```python
from build123d import *

# Parameters (mm, degrees)
F0_W     = 50
F0_H     = 50
F1_DEPTH = 15
F3_DEPTH = 60
F5_DEPTH = 5
F6_W     = 30
F6_H     = 5.4
F7_DEPTH = 30


with BuildPart() as f1:
    # F0 (on Top) → F1 (new body)
    with BuildSketch(Plane.XY):
        with Locations((25, -25)):
            Rectangle(F0_W, F0_H)
    extrude(amount=F1_DEPTH)

    # F2 (on face) → F3 (join)
    with BuildSketch(Plane.XY.offset(15)):
        Polygon((15, -30), (15, -50), (35, -50), (35, -30), (25, -17.510004), align=None)
    extrude(amount=F3_DEPTH)

    # F4 (on face) → F5 (cut)
    with BuildSketch(Plane(origin=(0, 0, 0), x_dir=(1, 0, 0), z_dir=(0, 0, -1))):
        Polygon((35, 50), (15, 50), (15, 30), (25, 17.510004), (35, 30), align=None)
    extrude(amount=-F5_DEPTH, mode=Mode.SUBTRACT)

    # F6 (on face) → F7 (cut)
    with BuildSketch(Plane.YZ.offset(50)):
        with Locations((-15, 7.7)):
            Rectangle(F6_W, F6_H)
    extrude(amount=-F7_DEPTH, mode=Mode.SUBTRACT)


solid = f1.part
```
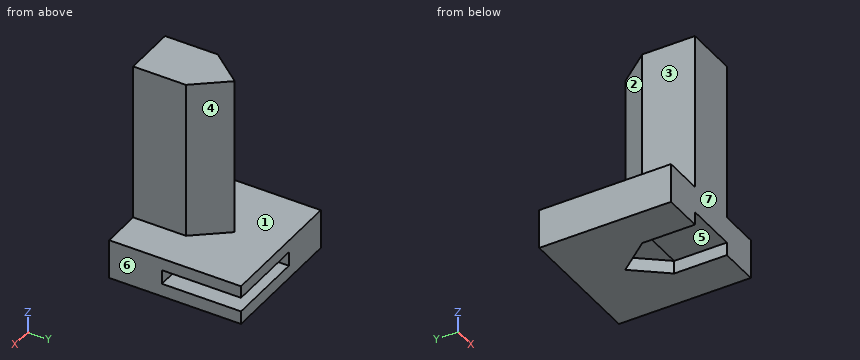
Design review of the part built by this model. Coordinates are the model's own, in mm. Face numbers are marked on the shaded views. A direction names the side the tool comes from. Give positions to 0.01 mm unless a question says otherwise; leave off trailing zeros. Write each loop counter-clockwise with the first axis right and the second up, starting at its lowest first coordinate (ties: lowest second). Pieces come first, ordered by that corner, then holes. Notation, with made-up numbers: (55, -17.75) -> (69, -17.75) arc R30 cw to (69, 16.25) -> close; hole circle Ø8 at (14.25, 70.25). An arc over 180 degrees is marked (long way). Answer in a Markdown table with one row per item.
(1) Consider section A-A (x = 26). State the section outline as (y, z) points.
Results:
| item | result |
|---|---|
| outline | (-50, 5) -> (-30, 5) -> (-30, 10.4) -> (0, 10.4) -> (0, 15) -> (-18.76, 15) -> (-18.76, 75) -> (-50, 75) -> close; (-18.76, 0) -> (0, 0) -> (0, 5) -> (-18.76, 5) -> close |
(2) Consider section C-C (y = -16). State the section outline as (x, z) points, then the cut area to 3 significant figures.
Results:
| item | result |
|---|---|
| outline | (0, 0) -> (50, 0) -> (50, 5) -> (20, 5) -> (20, 10.4) -> (50, 10.4) -> (50, 15) -> (0, 15) -> close |
| area | 588 mm2 |
(3) Consider section B-B (x = 40). State the section outline as (y, z) points.
Results:
| item | result |
|---|---|
| outline | (-50, 0) -> (0, 0) -> (0, 5) -> (-30, 5) -> (-30, 10.4) -> (0, 10.4) -> (0, 15) -> (-50, 15) -> close |
(4) To check wall thickness, follow probe 1 along Z at (x, y) = (28.5, -6.5); probe 2 along Y at (x, z) = (36, 9); probe 3 along X at (y, z) = (-36, 34). State the ranges of each line that lie inside material, in increasing order.
Results:
| item | result |
|---|---|
| probe 1 | 0 to 5, 10.4 to 15 |
| probe 2 | -50 to -30 |
| probe 3 | 15 to 35 |
(5) For the marked faces 1, 2, 3 and 4, list the 3-axis set-ups (+Z, -Z, +X, -X, +Y, -Y) from which the entire face can be reached by the end or side of a thin tool; tool diameter is ignored.
Results:
| item | result |
|---|---|
| face 1 | +Z, +Y |
| face 2 | +Z, -X, +Y |
| face 3 | +Z, -X, +Y, -Y |
| face 4 | +Z, +X, +Y |
(6) Consider section D-D (z = 40). State the section outline as (x, y) points.
Results:
| item | result |
|---|---|
| outline | (15, -50) -> (35, -50) -> (35, -30) -> (25, -17.51) -> (15, -30) -> close |
(7) Clearance check with flat-ended pins moving along their axes: pin 1 (5 mm diameter, centred on y = -38.5, z = 41, fed in from -X); pin 2 (8 mm diameter, centred on y = -14, z = 38.5, fed in from +X); pin 3 (4 mm diameter, centred on x = 30.5, y = -5.5, fed in from +Z). State where each tip first meets the part, or that it passes through.
Results:
| item | result |
|---|---|
| pin 1 | x = 15 |
| pin 2 | x = 25.39 |
| pin 3 | z = 15 |
(8) Mouldability with a two-part tool opening along X and no side actions: class the marked faces 5, 6 and 7 as +X half, -X half, draft (parallel to the pull), parting line (faces both ways), or undercut.
Results:
| item | result |
|---|---|
| face 5 | undercut |
| face 6 | +X half |
| face 7 | draft |
